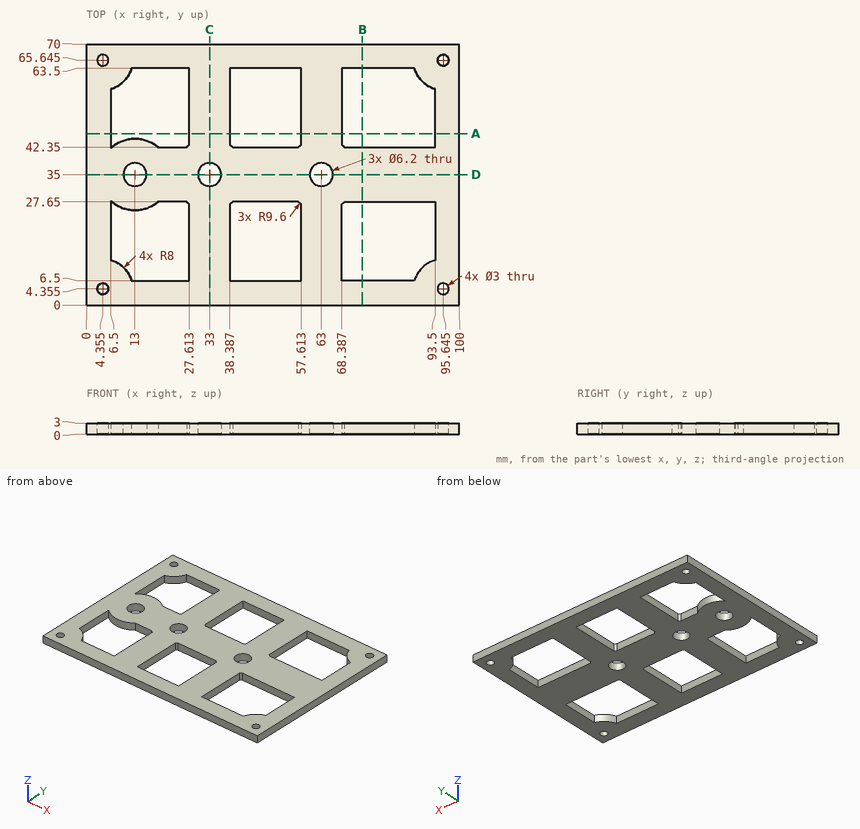
Study the drawing (mm; zero at the part's minimum x, y, z) and answer. Round coordinates to 2 decimals unless told otherwise and drop trailing zeros. Write each loop counter-clockwise with the first axis right and the second up, starting at its lowest first coordinate (ties: lowest second). Pieces come first, ordered by that corner, then holes.
1) A flat-ended cylindrical pin translates along its axis: P1, Ø8, axis at x = 50, y = 15.5, coming from the +Z side. Find the tip coordinate at first contact, or state that the pin passes through.
2) A cutting plane is placed at B-B on x = 74. Determine the outline of the cut face in (y, z).
3) A cutting plane is placed at D-D on y = 35. Determine the outline of the cut face in (x, z), and give its area (3 significant figures).
4) Consider probe 1 along Y at (x, z) = (86, 2.1); probe 2 along X at (y, z) = (52, 1.5); probe 3 along X at (y, z) = (59, 1.4) (1 decimal). Determine where each line is inside the solid, lowest interval first.
5) A cutting plane is placed at C-C on x = 33. Determine the outline of the cut face in (y, z).
6) A cutting plane is placed at A-A on y = 46. Determine the outline of the cut face in (x, z).
Entries:
1. P1: passes through
2. outline: (0, 0) - (6.5, 0) - (6.5, 3) - (0, 3) - close; (27.65, 0) - (42.35, 0) - (42.35, 3) - (27.65, 3) - close; (63.5, 0) - (70, 0) - (70, 3) - (63.5, 3) - close
3. outline: (0, 0) - (9.9, 0) - (9.9, 3) - (0, 3) - close; (16.1, 0) - (29.9, 0) - (29.9, 3) - (16.1, 3) - close; (36.1, 0) - (59.9, 0) - (59.9, 3) - (36.1, 3) - close; (66.1, 0) - (100, 0) - (100, 3) - (66.1, 3) - close
3. area: 244 mm2
4. probe 1: y = 0 to 6.5, 27.65 to 42.35, 63.5 to 70
4. probe 2: x = 0 to 6.5, 27.61 to 38.39, 57.61 to 68.39, 93.5 to 100
4. probe 3: x = 0 to 8.8, 27.6 to 38.4, 57.6 to 68.4, 91.2 to 100
5. outline: (0, 0) - (31.9, 0) - (31.9, 3) - (0, 3) - close; (38.1, 0) - (70, 0) - (70, 3) - (38.1, 3) - close
6. outline: (0, 0) - (6.5, 0) - (6.5, 3) - (0, 3) - close; (27.61, 0) - (38.39, 0) - (38.39, 3) - (27.61, 3) - close; (57.61, 0) - (68.39, 0) - (68.39, 3) - (57.61, 3) - close; (93.5, 0) - (100, 0) - (100, 3) - (93.5, 3) - close
